Study the drawing (mm; zero at the part's minimum x, y, z) and answer. A direction names the side the tool comes from. Round coordinates to 2 decimals unless told otherwise and drop trailing zeros. Loops run counter-clockwise (first coordinate to the right, second up) from the corner with the lowest first, then second, coordinate; pieces in that order, holes last. Notation, with made-up numbers: M 33.5,3 L 56.5,3 A11 cw 56.5,20 Z; hole C 39,-21 d5. An arc over 180 degrees is marked long. Put each result on its own line as item: value. Start each with the question number.
(1) Straight lines are drawn through the part: line 1 (Y direction, x = 5, z = 0.65); line 2 (Z direction, x = 3, y = 26.25); line 3 (Y direction, x = 5.5, z = 2.3). For each, find the intervals that lie inside material, in ascending order.
(2) Section D-D, the plane x = 7.75 is taken. Determine the outline of the cut face in (y, z).
(3) Flat-ended cylindrical pins translate along their axes: P1, Ø2, axis at x = 5, y = 25.4, coming from the -Z side (3 decimals); P2, Ø0.8, axis at x = 8, y = 7.5, coming from the +Z side; P3, Ø0.8, axis at x = 7.5, y = 4, coming from the -Z side; P4, Ø0.6, axis at y = 7.5, z = 3.5, coming from the -X side. Find the tip coordinate at first contact, or state that the pin passes through.
(4) Section A-A, the plane y = 6 is taken. Determine the outline of the cut face in (x, z).
(5) Section C-C, the plane y = 25.4 is taken. Determine the outline of the cut face in (x, z).
(6) Which of the six approach directions +Z, -Z, +X, -X, +Y, -Y give full straight-line access (tool end or side, diameter ignored) to the marked faces 1 and 2?
(7) Section B-B, the plane x = 5 is taken. Determine the outline of the cut face in (y, z).
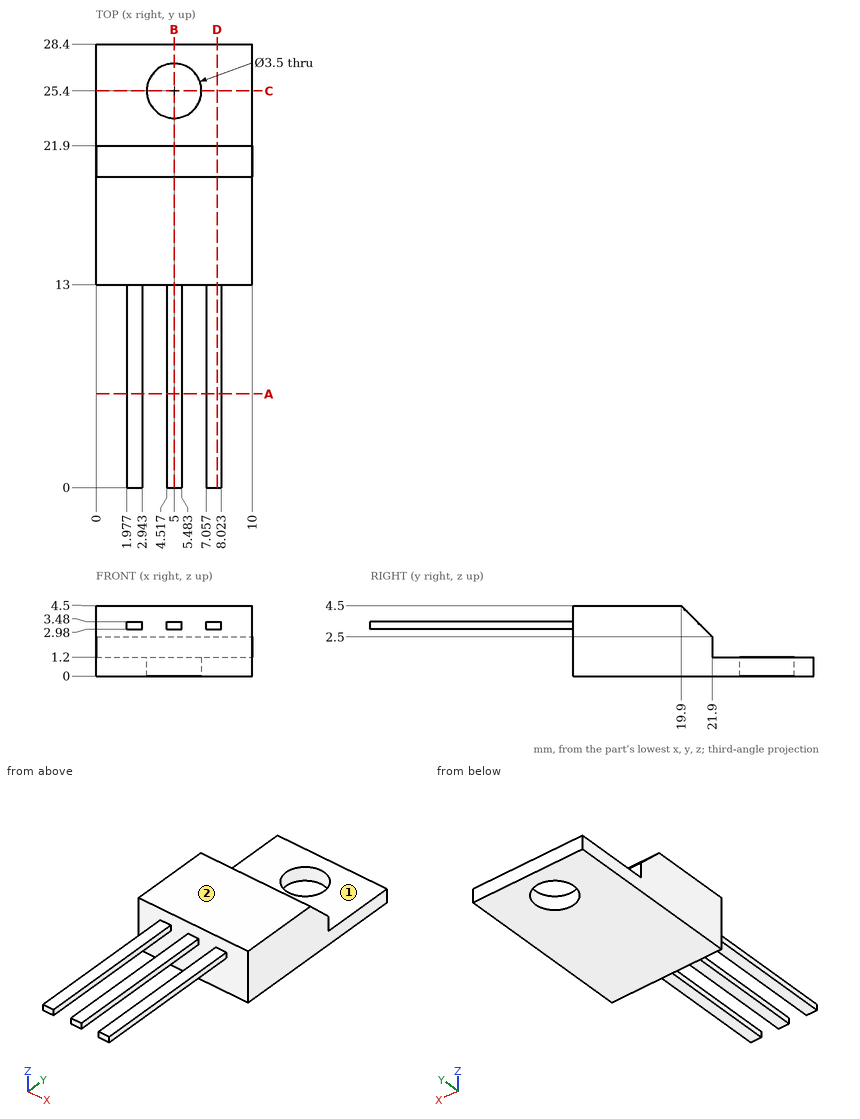
Recorded:
1. line 1: y = 13 to 23.65, 27.15 to 28.4
1. line 2: z = 0 to 1.2
1. line 3: y = 13 to 21.9
2. outline: M 0,2.98 L 13,2.98 L 13,0 L 28.4,0 L 28.4,1.2 L 21.9,1.2 L 21.9,2.5 L 19.9,4.5 L 13,4.5 L 13,3.48 L 0,3.48 Z
3. P1: passes through
3. P2: stops at z = 3.48
3. P3: stops at z = 2.98
3. P4: stops at x = 1.98
4. outline: M 1.98,2.98 L 2.94,2.98 L 2.94,3.48 L 1.98,3.48 Z; M 4.52,2.98 L 5.48,2.98 L 5.48,3.48 L 4.52,3.48 Z; M 7.06,2.98 L 8.02,2.98 L 8.02,3.48 L 7.06,3.48 Z
5. outline: M 0,0 L 3.25,0 L 3.25,1.2 L 0,1.2 Z; M 6.75,0 L 10,0 L 10,1.2 L 6.75,1.2 Z
6. face 1: +Z, +X, -X, +Y
6. face 2: +Z, +X, -X, +Y, -Y
7. outline: M 0,2.98 L 13,2.98 L 13,0 L 23.65,0 L 23.65,1.2 L 21.9,1.2 L 21.9,2.5 L 19.9,4.5 L 13,4.5 L 13,3.48 L 0,3.48 Z; M 27.15,0 L 28.4,0 L 28.4,1.2 L 27.15,1.2 Z
